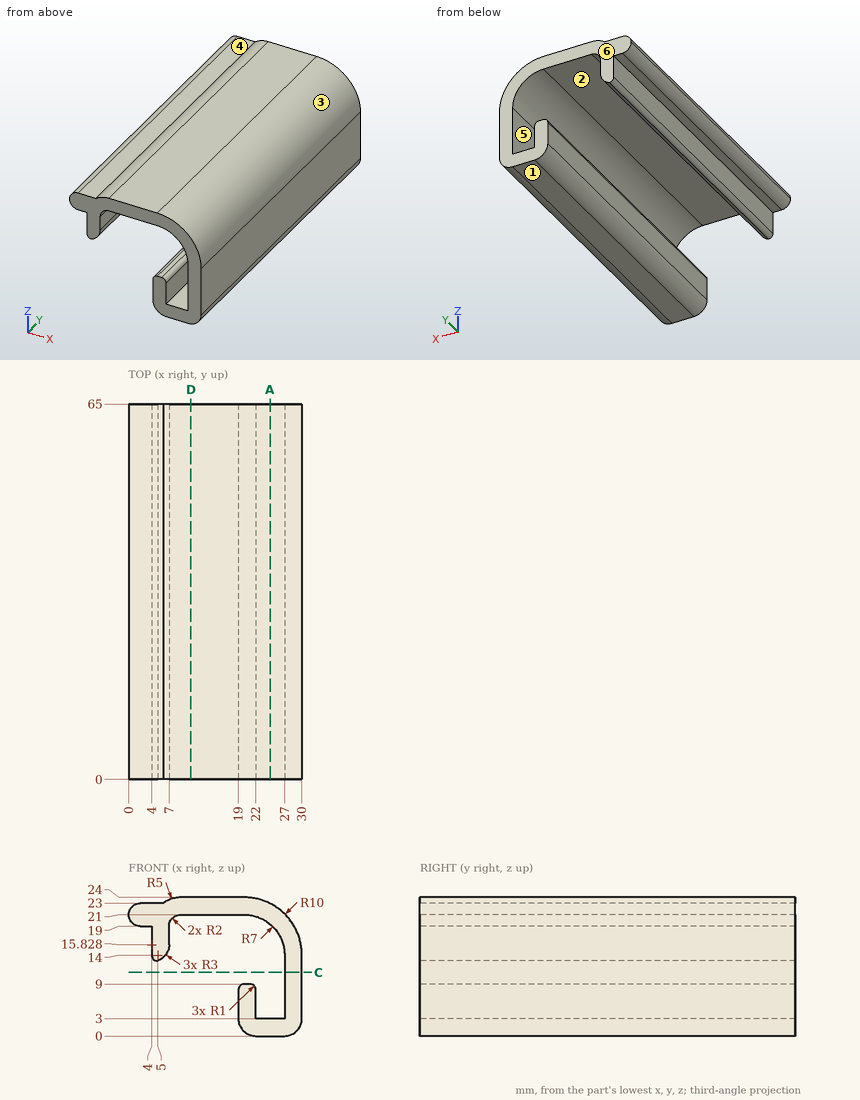
Design review of the part shown in the three views and the two pictorial views. Dimensions are in mm from the part's minimum x, y and z. A direction names the side the tool comes from. Round coordinates to 2 decimals unless told otherwise and drop trailing zeros. Loops run counter-clockwise (first coordinate to the right, second up) from the corner with the lowest first, then second, coordinate; pieces in that order, holes last. Notation, with made-up numbers: M -39.5,43.5 L -31.5,43.5 A26 cw -31.5,67.5 Z; hole C -23,-39.75 d9. An arc over 180 degrees is marked long. Answer as a JSON object with one key per item and string values.
Item 1: We need section C-C on z = 11. Give the boundary of the cut face in (x, y), and give its area (3 significant figures).
Answer sheet:
{"outline": "M 27,0 L 30,0 L 30,65 L 27,65 Z", "area": "195 mm^2"}
Item 2: Clearance check with flat-ended pins moving along their axes: P1, Ø12, axis at x = 10, y = 50.5, coming from the -Z side; P2, Ø2, axis at x = 20.5, y = 16, coming from the -Z side; P3, Ø1.5, axis at x = 6.5, y = 13, coming from the +Z side; P4, Ø2, axis at x = 6, z = 10.5, coming from the -Y side. State where each tip first meets the part, or that it passes through.
Answer sheet:
{"P1": "stops at z = 13", "P2": "stops at z = 0.04", "P3": "stops at z = 23.68", "P4": "passes through"}
Item 3: We need section A-A on x = 24.5. Give the boundary of the cut face in (y, z), and give its area (3 significant figures).
Answer sheet:
{"outline": "M 0,0 L 65,0 L 65,3 L 0,3 Z; M 0,19.36 L 65,19.36 L 65,22.93 L 0,22.93 Z", "area": "427 mm^2"}
Item 4: Wall thickness on L1, parallel to X at y = 30, z = 3.25; L2, parallel to X at y = 45, z = 12.75; L3, parallel to Z at x = 19.5, y = 18 (1 decimal): over which ranges is each line inside the solid? List them lowest first. Write a range as from..to.
Answer sheet:
{"L1": "x = 19..22, 27..30", "L2": "x = 27..30", "L3": "z = 1.3..8.9, 21..24"}
Item 5: Machinability: for the marked faces 4, 5 and 6, which of the approach directions +Z, -Z, +X, -X, +Y, -Y give a long, thin tool a straight path to every point of the face, cutting with its end or side? Answer none if there is none.
Answer sheet:
{"face 4": "+Z, -X, +Y, -Y", "face 5": "+Y, -Y", "face 6": "+Z, -Z, +X, -X, +Y"}
Item 6: We need section D-D on x = 10.75. Give the boundary of the cut face in (y, z).
Answer sheet:
{"outline": "M 0,21 L 65,21 L 65,24 L 0,24 Z"}
Item 7: The part is to be moulded in two halves that separate along X. For the marked faces 1, 2 and 3, say which applies: pulls with the +X half, pulls with the -X half, needs draft (parallel to the pull), parting line crosses it, or undercut.
Answer sheet:
{"face 1": "needs draft", "face 2": "undercut", "face 3": "pulls with the +X half"}
